Geometry check sheet. Reference: the model listing, model coordinates, mm. A direction names the side the tool comes from. Coordinates: 2 decimals unless noted, no trailing zeros. Write each loop counter-clockwise with the first axis right and the second up, starting at its lowest first coordinate (ties: lowest second). Pieces come first, ordered by that corner, then holes. Notation, with made-up numbers: (70.25, 44.5) -> (117.25, 44.5) arc R15 ccw to (117.25, 65.5) -> close; hole circle Ø11 at (81.25, 38.5). An arc over 180 degrees is marked (long way). Answer as CSV lines item,"result".
```python
from build123d import *

# Parameters (mm, degrees)
PAD_DEPTH = 2


with BuildPart() as part:
    # CopySketch004 → Pad (new body, symmetric)
    with BuildSketch(Plane.XY):
        with BuildLine():
            Line((-94.244626, 6.836694), (-74.920651, 10.704806))
            ThreePointArc((-63.603328, 11.826385), (-69.28971, 11.545305), (-74.920651, 10.704806))
            Line((-63.603328, 11.826385), (-42.55212, 11.826385))
            Line((-42.55212, 11.826385), (15.371862, 11.826385))
            ThreePointArc((15.371862, 11.826385), (31.195362, 15.106628), (44.410932, 24.406728))
            Line((44.410932, 24.406728), (55.444454, 36.175392))
            Line((55.444454, 36.175392), (100, 36.175392))
            Line((100, 36.175392), (100, 0))
            Line((100, 0), (16, 0))
            Line((16, -10), (16, 0))
            Line((2.15, -10), (16, -10))
            Line((2.15, 1.647389), (2.15, -10))
            Line((-2.15, 1.647389), (2.15, 1.647389))
            Line((-2.15, -10), (-2.15, 1.647389))
            Line((-16, -10), (-2.15, -10))
            Line((-16, 0), (-16, -10))
            Line((-16, 0), (-100, 0))
            ThreePointArc((-94.244626, 6.836694), (-98.319024, 4.425781), (-100, 0))
        make_face()
    extrude(amount=PAD_DEPTH, both=True)


solid = part.part
```
Item 1: Thickness scan on probe 1 along X at (y, z) = (-0.5, 0.35); probe 2 along Y at (x, z) = (11, 1.3); probe 3 along Y at (x, z) = (-47.5, 0). Record the ranges inside material, lowest first.
Responses:
probe 1,"x = -16 to -2.15, 2.15 to 16"
probe 2,"y = -10 to 11.83"
probe 3,"y = 0 to 11.83"
Item 2: Cross-section at C-C, the plane x = 65.5. Record the cut outline in (y, z).
Responses:
outline,"(0, -2) -> (36.18, -2) -> (36.18, 2) -> (0, 2) -> close"
Item 3: Cross-section at A-A, the plane y = -5.5. Record the cut outline in (x, z), plus the area to 3 significant figures.
Responses:
outline,"(-16, -2) -> (-2.15, -2) -> (-2.15, 2) -> (-16, 2) -> close; (2.15, -2) -> (16, -2) -> (16, 2) -> (2.15, 2) -> close"
area,"111 mm2"
Item 4: Cross-section at D-D, the plane y = 8.5. Record the cut outline in (x, z).
Responses:
outline,"(-85.94, -2) -> (100, -2) -> (100, 2) -> (-85.94, 2) -> close"
Item 5: Set-up check for faces 4 (the flat face through (-2.15, -4, 0)), 5 (the flat face through (16, -5, 0)), 6 (the flat face through (-25, 11.826, 0)): record each of +Z, -Z, +X, -X, +Y, -Y from which the full face is reachable in a straight line by a thin tool's end or side.
Responses:
face 4,"+Z, -Z, -Y"
face 5,"+Z, -Z, +X, -Y"
face 6,"+Z, -Z, -X, +Y"
Item 6: Cross-section at B-B, the plane z = 1.2. Record the cut outline in (x, y), plus the area to 3 significant figures.
Responses:
outline,"(-100, 0) -> (-16, 0) -> (-16, -10) -> (-2.15, -10) -> (-2.15, 1.65) -> (2.15, 1.65) -> (2.15, -10) -> (16, -10) -> (16, 0) -> (100, 0) -> (100, 36.18) -> (55.44, 36.18) -> (44.41, 24.41) arc R39.81 cw to (15.37, 11.83) -> (-63.6, 11.83) arc R57.66 ccw to (-74.92, 10.7) -> (-94.24, 6.84) arc R7.16 ccw to start"
area,"3,930 mm2"
Item 7: Depth check by flat-ended pin: pin 1 Ø1.2 at (y, z) = (-3.5, 0.5) entering from -X; pin 2 Ø1 at (y, z) = (30, 1) entering from -X; pin 3 Ø1 at (y, z) = (23, 0) entering from -X; pin 4 Ø8 at (x, y) = (-75, 14) entering from -Z. Enter the tip coordinate at first touch or a pass-through.
Responses:
pin 1,"stops at x = -16"
pin 2,"stops at x = 49.19"
pin 3,"stops at x = 42.5"
pin 4,"stops at z = -2"
Item 8: Release check for a two-part mould opening along X. For faces 1 (the flat face through (46, 13, 2)), 2 (the flat face through (-16, -5, 0)), 3 (the flat face through (0, 1.647, 0)) record: +X half, -X half, draft (parallel to the pull), parting line (faces both ways), or undercut.
Responses:
face 1,"draft"
face 2,"-X half"
face 3,"undercut"
